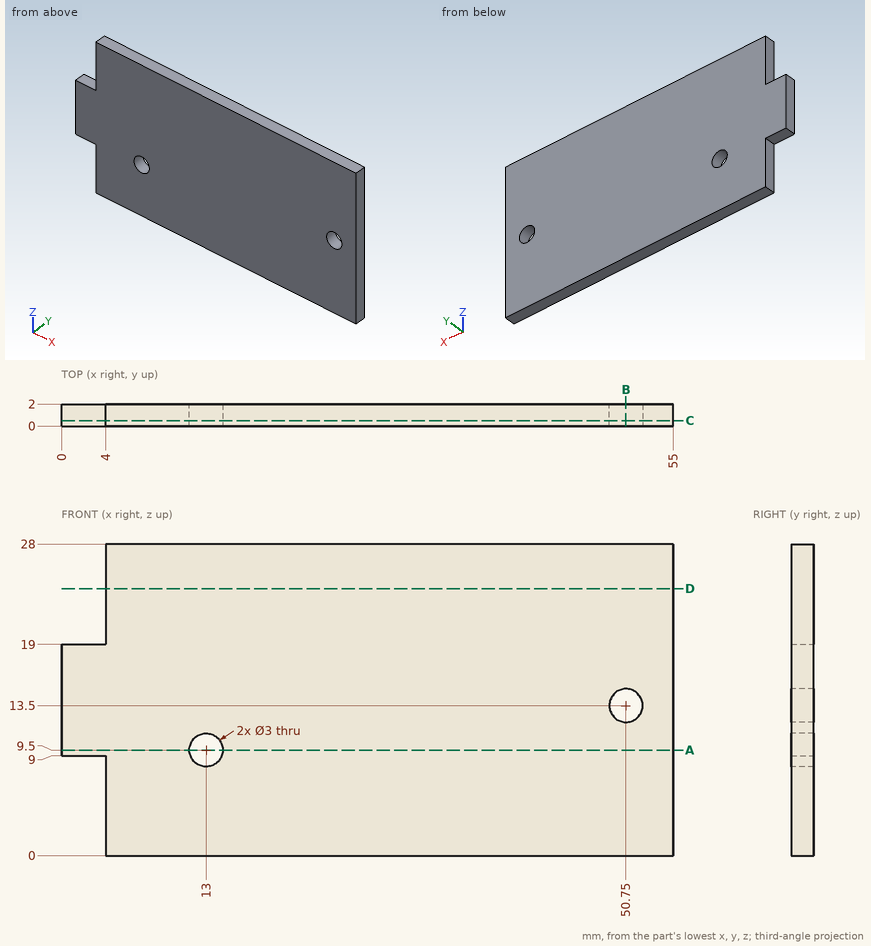
Check sheet for the drawn part. Datum: minimum x, y, z corner. Units: mm. Round coordinates to 2 decimals unless told otherwise and drop trailing zeros. Write each loop counter-clockwise with the first axis right and the second up, starting at its lowest first coordinate (ties: lowest second). Pieces come first, ordered by that corner, then holes. Notation, with made-up numbers: (-19, -27.5) -> (22, -27.5) arc R10 cw to (22, -13.5) -> close; hole circle Ø5 at (29.5, -36). An arc over 180 degrees is marked (long way). Write each question's results on one line, items separated by ' | '.
Q1. Sectioned sample at C-C, the plane y = 0.5. Record the boundary of the cut face in (x, z).
Derived:
outline: (0, 9) -> (4, 9) -> (4, 0) -> (55, 0) -> (55, 28) -> (4, 28) -> (4, 19) -> (0, 19) -> close; hole circle Ø3 at (13, 9.5); hole circle Ø3 at (50.75, 13.5)
Q2. Sectioned sample at A-A, the plane z = 9.5. Record the boundary of the cut face in (x, y).
Derived:
outline: (0, 0) -> (11.5, 0) -> (11.5, 2) -> (0, 2) -> close; (14.5, 0) -> (55, 0) -> (55, 2) -> (14.5, 2) -> close
Q3. Go/stop test with flat-tipped pins: pin 1 Ø1 at (y, z) = (0.5, 22.5) entering from -X; pin 2 Ø2.5 at (x, z) = (13, 9.5) entering from +Y; pin 3 Ø0.6 at (x, y) = (1.5, 1) entering from -Z. Record where each tip stops, or that it passes through.
Derived:
pin 1: stops at x = 4 | pin 2: passes through | pin 3: stops at z = 9
Q4. Thickness scan on probe 1 along X at (y, z) = (0.75, 13.5); probe 2 along Z at (x, y) = (13, 1.4); probe 3 along Z at (x, y) = (50.75, 1.3). Record the ranges inside material, lowest first.
Derived:
probe 1: x = 0 to 49.25, 52.25 to 55 | probe 2: z = 0 to 8, 11 to 28 | probe 3: z = 0 to 12, 15 to 28
Q5. Sectioned sample at D-D, the plane z = 24. Record the boundary of the cut face in (x, y).
Derived:
outline: (4, 0) -> (55, 0) -> (55, 2) -> (4, 2) -> close
Q6. Sectioned sample at B-B, the plane x = 50.75. Record the boundary of the cut face in (y, z).
Derived:
outline: (0, 0) -> (2, 0) -> (2, 12) -> (0, 12) -> close; (0, 15) -> (2, 15) -> (2, 28) -> (0, 28) -> close
